from build123d import *

# Parameters (mm, degrees)
F0_W      = 50
F0_H      = 50
F1_DEPTH  = 50
F4_DEPTH  = 10
F5_SIZE   = 10
F6_W      = 10
F6_H      = 40
F8_DEPTH  = 40
F9_R      = 10
F11_DEPTH = 6


with BuildPart() as f1:
    # F0 (on Top) → F1 (new body)
    with BuildSketch(Plane.XY):
        with Locations((-6.196748, 1.000199)):
            Rectangle(F0_W, F0_H)
    extrude(amount=F1_DEPTH)

    # F3 (on face) → F4 (cut)
    with BuildSketch(Plane.XY.offset(50)):
        with BuildLine():
            ThreePointArc((-31.196748, -8.999801), (-20.590146, -13.393199), (-16.196748, -23.999801))
            Line((-16.196748, -23.999801), (-6.196748, -23.999801))
            Line((-6.196748, -23.999801), (-6.196748, 1.000199))
            Line((-6.196748, 1.000199), (-31.196748, 1.000199))
            Line((-31.196748, 1.000199), (-31.196748, -8.999801))
        make_face()
    extrude(amount=-F4_DEPTH, mode=Mode.SUBTRACT)

    # F5
    f5_edges = [f1.edges().sort_by_distance(p)[0] for p in [
        (-6.196748, 1.000199, 45),
    ]]
    chamfer(f5_edges, length=F5_SIZE)

    # F6 (on face) → F8 (cut, through all)
    with BuildSketch(Plane.XY.offset(50)):
        with Locations((7.803252, -3.999801)):
            Rectangle(F6_W, F6_H)
    extrude(amount=-F8_DEPTH, mode=Mode.SUBTRACT)

    # F9
    f9_edges = [f1.edges().sort_by_distance(p)[0] for p in [
        (7.803252, 16.000199, 10),
    ]]
    fillet(f9_edges, radius=F9_R)

    # F10 (on face) → F11 (cut)
    with BuildSketch(Plane.YZ.offset(18.803252)):
        Polygon((-3.999801, 50), (-23.999801, 50), (-23.999801, 30), align=None)
    extrude(amount=-F11_DEPTH, mode=Mode.SUBTRACT)

    # F12 (on face) → F13 (revolve, cut)
    with BuildSketch(Plane.XZ.offset(23.999801)):
        Polygon((-6.196748, 20), (-31.196748, 50), (-31.196748, 0), (-6.196748, 0), align=None)
    revolve(axis=Axis((-31.196748, -23.999801, 25), (0, 0, 1)), mode=Mode.SUBTRACT)


solid = f1.part
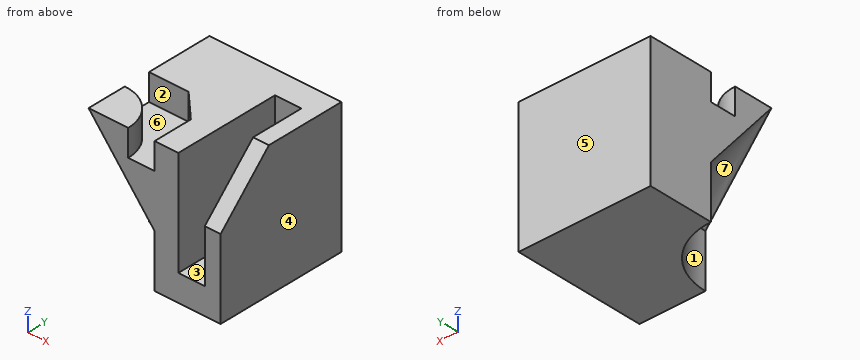
Can you work these out from the model? Positions are in its coordinate system, mm. Face numbers are marked on the shaded views. A direction names the side the tool comes from. Give positions to 0.01 mm unless a question says otherwise; leave off trailing zeros. Order: outer loops, then holes, each group sorted by start corner. A loop starts at its lowest first (then second) coordinate and runs counter-clockwise, first axis right, second up. Notation, with made-up numbers: M 12.25,55 L 20.25,55 A19 cw 20.25,73 Z; hole C 34,12 d2. An arc over 180 degrees is marked long. Use a Markdown table: item, result. Add a question column.
Item 1: If I drill on L1, parallel to X at y = 4, z = 22.5; L2, parallel to Z at x = 8, y = -9; L3, parallel to Z at x = -14.5, y = -2, over which ranges is the centre line in solid material (lowest first)? Write a range as [from, to].
Item 2: We'd pull the mould along X, two halves only. Please class the marked faces 4, 5, 6 and 7: +X half, -X half, draft (parallel to the pull), parting line (faces both ways), or undercut.
Item 3: For the marked faces 1, 2 and 3, which set-ups out of +Z, -Z, +X, -X, +Y, -Y let a thin tool reach every point of the face, with its end or its side?
Item 4: Suppose I cut it at B-B (x = 4). List the corners of the cut face in (y, z) for me, then the cut area to 3 significant figures.
Item 5: Suppose I cut it at D-D (z = 25.5). List the corners of the cut face in (x, y) for me, then the cut area to 3 significant figures.
Item 6: Suppose I cut it at C-C (z = 16). List the corners of the cut face in (x, y) for me.
Item 7: Will these pins go through, and if not, where does the flat tip stop? pin 1 (5 mm diameter, centred on x = 5.5, z = 34.5, fed in from -Y); pin 2 (6 mm diameter, centred on x = -17, z = 6.5, fed in from -Y); pin 3 (5 mm diameter, centred on x = 6.5, y = -16, fed in from +Z).
Item 8: Suppose I cut it at A-A (y = 2). List the corners of the cut face in (x, z) for me, then the cut area to 3 significant figures.
Answer sheet:
| question | item | result |
|---|---|---|
| 1 | L1 | x = [-31.2, 2.8], [12.8, 18.8] |
| 1 | L2 | z = [0, 10] |
| 1 | L3 | z = [0, 40] |
| 2 | face 4 | +X half |
| 2 | face 5 | draft |
| 2 | face 6 | undercut |
| 2 | face 7 | -X half |
| 3 | face 1 | -Z, -X, -Y |
| 3 | face 2 | +Z, -X |
| 3 | face 3 | +Z, -Y |
| 4 | outline | M -24,0 L 26,0 L 26,50 L 16,50 L 16,20 A10 cw 6,10 L -24,10 Z |
| 4 | area | 921 mm² |
| 5 | outline | M -31.2,-3.58 A20.42 cw -10.78,-24 L 2.8,-24 L 2.8,16 L 12.8,16 L 12.8,-24 L 18.8,-24 L 18.8,26 L -31.2,26 Z |
| 5 | area | 1,770 mm² |
| 6 | outline | M -31.2,1 A25 cw -6.2,-24 L 2.8,-24 L 2.8,15.17 L 12.8,15.17 L 12.8,-24 L 18.8,-24 L 18.8,26 L -31.2,26 Z |
| 7 | pin 1 | stops at y = 16 |
| 7 | pin 2 | stops at y = -5.85 |
| 7 | pin 3 | stops at z = 10 |
| 8 | outline | M -31.2,0 L 18.8,0 L 18.8,50 L 12.8,50 L 12.8,10 L 2.8,10 L 2.8,50 L -31.2,50 Z |
| 8 | area | 2,100 mm² |
